Read the model definition and answer for the solid it produces. Units are mm, in the model's axes. Face numbers are marked on the shaded views. A direction names the side the tool comes from. Give positions to 0.01 mm unless a question says otherwise; leave off trailing zeros. Order: outer loops, then holes, each group sorted by start corner. A loop starts at its lowest first (then second) coordinate and runs counter-clockwise, first axis right, second up. Notation, with made-up numbers: (-14.5, 47) -> (17.5, 47) arc R30 cw to (17.5, 84) -> close; hole circle Ø11 at (7, 55.25). An arc over 180 degrees is marked (long way). Answer as CSV lines item,"result". Start each with the question number.
1) Straight lines are drawn through the part: L1, parallel to Y at x = 0.05, z = 13; L2, parallel to X at y = 0.4, z = 6.25; L3, parallel to Y at x = -1, z = 3. For each, find the intervals that lie inside material, in ascending order. Write a range as from..to.
2) For the marked faces 1 and 2, determine the directions among +Z, -Z, +X, -X, +Y, -Y from which every point of the face is accessible in a straight line to the end or side of a thin tool.
3) Flat-ended cylindrical pins translate along their axes: pin 1 Ø1.5 at (x, y) = (-0.5, -1) entering from -Z; pin 2 Ø1 at (y, z) = (-2, 12) entering from -X; pin 3 Ø1 at (y, z) = (2, 9) entering from +X; pin 4 Ø1.5 at (y, z) = (-1, 12) entering from -X. Find the tip coordinate at first contact, or state that the pin passes through.
4) Find section A-A (z = 4.25). Determine the outline of the cut face in (x, y).
5) Find section B-B (z = 16). Determine the outline of the cut face in (x, y) (3 decimals), and give its area (3 significant figures).
```python
from build123d import *

# Parameters (mm, degrees)
SKETCH_1_R      = 2.45
EXTRUDE_1_DEPTH = 15
SKETCH_2_R      = 2.475
EXTRUDE_2_DEPTH = 3
FILLET_1_R      = 0.3
FILLET_2_R      = 0.3


with BuildPart() as part:
    # 스케치1 → 보스-돌출1 (new body)
    with BuildSketch(Plane.XY):
        Circle(SKETCH_1_R)
    extrude(amount=EXTRUDE_1_DEPTH)

    # 스케치2 → 보스-돌출2 (add)
    with BuildSketch(Plane.XY.offset(15)):
        Circle(SKETCH_2_R)
    extrude(amount=EXTRUDE_2_DEPTH)

    # 필렛1
    fillet_1_edges = [part.edges().sort_by_distance(p)[0] for p in [
        (-2.475, 0, 18),
    ]]
    fillet(fillet_1_edges, radius=FILLET_1_R)

    # 필렛2
    fillet_2_edges = [part.edges().sort_by_distance(p)[0] for p in [
        (-2.45, 0, 0),
    ]]
    fillet(fillet_2_edges, radius=FILLET_2_R)


solid = part.part
```
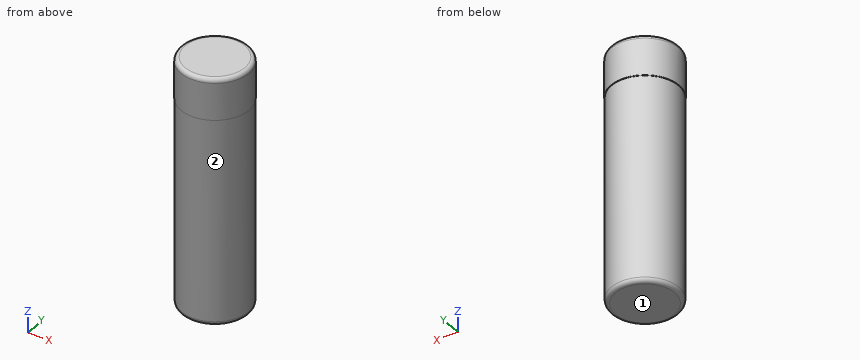
Findings below:
1,L1,"-2.45..2.45"
1,L2,"-2.42..2.42"
1,L3,"-2.24..2.24"
2,face 1,"-Z, +X, -X, +Y, -Y"
2,face 2,"-Z"
3,pin 1,"z = 0"
3,pin 2,"x = -1.94"
3,pin 3,"x = 1.94"
3,pin 4,"x = -2.44"
4,outline,"circle Ø4.9 at (0, 0)"
5,outline,"circle Ø4.95 at (0, 0)"
5,area,"19.2 mm²"
